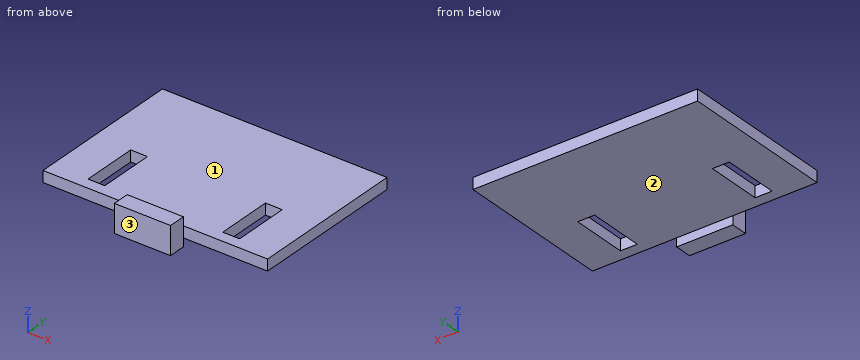
```python
from build123d import *

# Parameters (mm, degrees)
SKETCH1_W               = 40
SKETCH1_H               = 28
BOSS_EXTRUDE1_DEPTH     = 2
CUT_EXTRUDE1_DEPTH      = 25.494897428
CUT_EXTRUDE1_DEPTH_BACK = 25.494897428
SKETCH2_W               = 3
SKETCH2_H               = 10
SKETCH5_W               = 10
SKETCH5_H               = 5
BOSS_EXTRUDE2_DEPTH     = 3


with BuildPart() as part:
    # Sketch1 → Boss-Extrude1 (new body)
    with BuildSketch(Plane.XY):
        Rectangle(SKETCH1_W, SKETCH1_H)
    extrude(amount=BOSS_EXTRUDE1_DEPTH)

    # Sketch2 → Cut-Extrude1 (cut, two sides: drawn at the far end of the back side and taken through both)
    with BuildSketch(Plane.XY.offset(2).offset(-CUT_EXTRUDE1_DEPTH_BACK)):
        with Locations((-12, -7)):
            Rectangle(SKETCH2_W, SKETCH2_H)
        with Locations((12, -7)):
            Rectangle(SKETCH2_W, SKETCH2_H)
    extrude(amount=CUT_EXTRUDE1_DEPTH + CUT_EXTRUDE1_DEPTH_BACK, mode=Mode.SUBTRACT)

    # Sketch5 → Boss-Extrude2 (add)
    with BuildSketch(Plane(origin=(0, -14, 0), x_dir=(-1, 0, 0), z_dir=(0, -1, 0))):
        with Locations((0, -1)):
            Rectangle(SKETCH5_W, SKETCH5_H)
    extrude(amount=BOSS_EXTRUDE2_DEPTH)


solid = part.part
```
Read the model definition and answer for the solid it produces. Units are mm, in the model's axes. Face numbers are marked on the shaded views. Coordinates: 2 decimals unless noted, no trailing zeros. Loops run counter-clockwise (first coordinate to the right, second up) from the corner with the lowest first, then second, coordinate; pieces in that order, holes last.
(1) The part is cut by section B-B (y = -6.5). Determine the outline of the cut face in (x, z), and give its area (3 significant figures).
Solution:
outline: (-20, 0) - (-13.5, 0) - (-13.5, 2) - (-20, 2) - close; (-10.5, 0) - (10.5, 0) - (10.5, 2) - (-10.5, 2) - close; (13.5, 0) - (20, 0) - (20, 2) - (13.5, 2) - close
area: 68.0 mm2
(2) Consider line 1 along X through (y, z) = (-4.5, 1.05); line 2 along X through (y, z) = (-14.5, 2.85); line 3 along Z through (x, y) = (-18, -1). Determine where each line is inside the solid, lowest interval first.
Solution:
line 1: x = -20 to -13.5, -10.5 to 10.5, 13.5 to 20
line 2: x = -5 to 5
line 3: z = 0 to 2
(3) The mould has two halves that part along Z. Classify the marked faces 1, 2 and 3: released by +Z, released by -Z, zero draft, split by the parting line, or undercut.
Solution:
face 1: released by +Z
face 2: released by -Z
face 3: zero draft
(4) The part is cut by section A-A (x = 12.5). Determine the outline of the cut face in (y, z), and give its area (3 significant figures).
Solution:
outline: (-14, 0) - (-12, 0) - (-12, 2) - (-14, 2) - close; (-2, 0) - (14, 0) - (14, 2) - (-2, 2) - close
area: 36.0 mm2
(5) The part is cut by section C-C (x = 1). Determine the outline of the cut face in (y, z), and give its area (3 significant figures).
Solution:
outline: (-17, -1.5) - (-14, -1.5) - (-14, 0) - (14, 0) - (14, 2) - (-14, 2) - (-14, 3.5) - (-17, 3.5) - close
area: 71.0 mm2
(6) Flat-ended cylindrical pins translate along their axes: pin 1 Ø2 at (x, z) = (-12, 0) entering from -Y; pin 2 Ø1.5 at (y, z) = (-1.5, -0.5) entering from +X; pin 3 Ø3 at (x, y) = (-10.5, -5.5) entering from +Z; pin 4 Ø0.8 at (x, z) = (-0.5, 2.5) entering from +Y. Find the tip coordinate at first contact, or state that the pin passes through.
Solution:
pin 1: stops at y = -14
pin 2: stops at x = 20
pin 3: stops at z = 2
pin 4: stops at y = -14
(7) The part is cut by section D-D (y = -1). Determine the outline of the cut face in (x, z).
Solution:
outline: (-20, 0) - (20, 0) - (20, 2) - (-20, 2) - close
